from build123d import *

# Parameters (mm, degrees)
F0_R            = 100
F1_DEPTH        = 25
F3_DEPTH        = 25
F3_COPIES_COUNT = 20
F4_SIZE         = 2
F5_R            = 5
F6_R            = 90
F7_DEPTH        = 5


# Not quite as in the source:
# - a pattern or mirror of a feature is missing from the dataset's text; its kind, count and spacing are read off the source's solid


with BuildPart() as f1:
    # F0 (on Front) → F1 (new body)
    with BuildSketch(Plane.XZ):
        Circle(F0_R)
    extrude(amount=F1_DEPTH)

    # F2 (on Front) → F3 (join)
    with BuildSketch(Plane.XZ):
        Polygon((4.5, 120), (-4.5, 120), (-9.9931095726, 99.4994359837), (9.9931095726, 99.4994359837), align=None)
    f3 = extrude(amount=F3_DEPTH)

    # F3_copies: F3 ×20 about axis
    f3_copies_axis = Axis((0, 0, 0), (0, 1, 0))
    for i in range(1, F3_COPIES_COUNT):
        add(f3.rotate(f3_copies_axis, i * 360 / F3_COPIES_COUNT))

    # F4
    f4_edges = [f1.edges().sort_by_distance(p)[0] for p in [
        (4.5, -12.5, 120),
        (-4.5, -12.5, 120),
        (-32.802285, -12.5, 115.517358),
        (115.517358, -12.5, 32.802285),
        (120, -12.5, 4.5),
        (120, -12.5, -4.5),
        (115.517358, -12.5, -32.802285),
        (112.736205, -12.5, -41.361794),
        (99.727073, -12.5, -66.893654),
        (94.437006, -12.5, -74.174807),
        (74.174807, -12.5, -94.437006),
        (66.893654, -12.5, -99.727073),
        (41.361794, -12.5, -112.736205),
        (32.802285, -12.5, -115.517358),
        (4.5, -12.5, -120),
        (-4.5, -12.5, -120),
        (-32.802285, -12.5, -115.517358),
        (-41.361794, -12.5, -112.736205),
        (-66.893654, -12.5, -99.727073),
        (-74.174807, -12.5, -94.437006),
        (-94.437006, -12.5, -74.174807),
        (-99.727073, -12.5, -66.893654),
        (-112.736205, -12.5, -41.361794),
        (-115.517358, -12.5, -32.802285),
        (-120, -12.5, -4.5),
        (-120, -12.5, 4.5),
        (-115.517358, -12.5, 32.802285),
        (-112.736205, -12.5, 41.361794),
        (-99.727073, -12.5, 66.893654),
        (-94.437006, -12.5, 74.174807),
        (-74.174807, -12.5, 94.437006),
        (-66.893654, -12.5, 99.727073),
        (32.802285, -12.5, 115.517358),
        (41.361794, -12.5, 112.736205),
        (66.893654, -12.5, 99.727073),
        (74.174807, -12.5, 94.437006),
        (94.437006, -12.5, 74.174807),
        (99.727073, -12.5, 66.893654),
        (112.736205, -12.5, 41.361794),
        (-41.361794, -12.5, 112.736205),
    ]]
    chamfer(f4_edges, length=F4_SIZE)

    # F5
    f5_edges = [f1.edges().sort_by_distance(p)[0] for p in [
        (9.99311, -12.5, 99.499436),
        (-9.99311, -12.5, 99.499436),
        (97.717628, -12.5, 21.243005),
        (99.499436, -12.5, 9.99311),
        (91.541546, -12.5, 40.251029),
        (86.370537, -12.5, 50.399706),
        (99.499436, -12.5, -9.99311),
        (97.717628, -12.5, -21.243005),
        (74.622932, -12.5, 66.568897),
        (66.568897, -12.5, 74.622932),
        (91.541546, -12.5, -40.251029),
        (86.370537, -12.5, -50.399706),
        (50.399706, -12.5, 86.370537),
        (40.251029, -12.5, 91.541546),
        (74.622932, -12.5, -66.568897),
        (66.568897, -12.5, -74.622932),
        (21.243005, -12.5, 97.717628),
        (50.399706, -12.5, -86.370537),
        (40.251029, -12.5, -91.541546),
        (-21.243005, -12.5, 97.717628),
        (21.243005, -12.5, -97.717628),
        (9.99311, -12.5, -99.499436),
        (-40.251029, -12.5, 91.541546),
        (-50.399706, -12.5, 86.370537),
        (-9.99311, -12.5, -99.499436),
        (-21.243005, -12.5, -97.717628),
        (-66.568897, -12.5, 74.622932),
        (-74.622932, -12.5, 66.568897),
        (-40.251029, -12.5, -91.541546),
        (-50.399706, -12.5, -86.370537),
        (-86.370537, -12.5, 50.399706),
        (-91.541546, -12.5, 40.251029),
        (-66.568897, -12.5, -74.622932),
        (-74.622932, -12.5, -66.568897),
        (-97.717628, -12.5, 21.243005),
        (-99.499436, -12.5, 9.99311),
        (-86.370537, -12.5, -50.399706),
        (-91.541546, -12.5, -40.251029),
        (-99.499436, -12.5, -9.99311),
        (-97.717628, -12.5, -21.243005),
    ]]
    fillet(f5_edges, radius=F5_R)

    # F6 (on face) → F7 (cut)
    with BuildSketch(Plane.XZ.offset(25)):
        Circle(F6_R)
    extrude(amount=-F7_DEPTH, mode=Mode.SUBTRACT)


solid = f1.part
Source: CAD feature listing. Evaluate the final solid. Frame: model axes, mm. A direction names the side the tool comes from. Round coordinates to 2 decimals unless told otherwise and drop trailing zeros. Order: outer loops, then holes, each group sorted by start corner. A loop starts at its lowest first (then second) coordinate and runs counter-clockwise, first axis right, second up. Notation, with made-up numbers: (-17, 25) - (25, 25) arc R21 cw to (25, 36) - close; hole circle Ø10 at (-16, 2.25). An arc over 180 degrees is marked (long way). Use a Markdown table: item, result. Add a question column.
1. First-contact query: pin 1 (1 mm diameter, centred on x = 55.5, z = -49.5, fed in from -Y); pin 2 (2 mm diameter, centred on x = -50.5, y = -18, fed in from +Z); pin 3 (3 mm diameter, centred on y = -9.5, z = -88.5, fed in from +X); pin 4 (5 mm diameter, centred on x = -4.5, z = 8.5, fed in from +Y). Flat tips, straight axial feed; report the tip coordinate or a pass-through.
2. Section query B-B (z = -84.5). Return the cut outline in (x, y).
3. Line query: probe 1 along Z at (x, y) = (0, -23.9); probe 2 along X at (y, z) = (-2.75, -108); probe 3 along X at (y, z) = (-21.5, 107.5). Output: solid intervals per line, ascending.
4. Set-up query: faces 1 (the flat face through (-107.29, -12.32, 27.46)), 2 (the cylindrical face through (-67.566, -12.675, 74.94)), 3 (the flat face through (93.417, -12.325, 59.101)), 4 (the flat face through (-27.46, -12.32, -107.29)), 5 (the flat face through (85.28, -12.32, 70.66)). Return all of +Z, -Z, +X, -X, +Y, -Y with unobstructed straight access to the full face (end or side cutting, diameter ignored); none if empty.
5. Section query A-A (z = -56). Return the cut outline in (x, y).
6. Mould query, pull axis X, two halves, no side actions, for faces 6 (the flat face through (107.108, -12.325, 27.341)), 7 (the flat face through (59.101, -12.325, -93.417)), 8 (the cylindrical face through (-87.41, -12.68, -50.31)). Classes: +X half, -X half, draft (parallel to the pull), parting line (faces both ways), or undercut.
Derived:
| question | item | result |
|---|---|---|
| 1 | pin 1 | y = -20 |
| 1 | pin 2 | z = 87.66 |
| 1 | pin 3 | x = 72.47 |
| 1 | pin 4 | y = 0 |
| 2 | outline | (-70.36, -25) - (-30.98, -25) - (-30.98, -20) - (30.98, -20) - (30.98, -25) - (70.36, -25) - (70.36, 0) - (-70.36, 0) - close |
| 3 | probe 1 | -120 to -90, 90 to 120 |
| 3 | probe 2 | -41.11 to -27.92, -7.72 to 7.72, 27.92 to 41.11 |
| 3 | probe 3 | -41.09 to -27.6, -7.85 to 7.85, 27.6 to 41.09 |
| 4 | face 1 | -X, +Y, -Y |
| 4 | face 2 | +Y, -Y |
| 4 | face 3 | +X, +Y, -Y |
| 4 | face 4 | -Z, +Y, -Y |
| 4 | face 5 | +Z, +Y, -Y |
| 5 | outline | (-90.91, -25) - (-70.46, -25) - (-70.46, -20) - (70.46, -20) - (70.46, -25) - (90.91, -25) - (90.91, 0) - (-90.91, 0) - close |
| 6 | face 6 | +X half |
| 6 | face 7 | undercut |
| 6 | face 8 | -X half |
